Input: part model. Units: mm. Frame: model coordinates. Round coordinates to 2 decimals unless told otherwise and drop trailing zeros. Loops run counter-clockwise (first coordinate to the right, second up) from the corner with the lowest first, then second, coordinate; pieces in that order, holes last.
1) Ray query, line 1 along Y through (x, z) = (-118.6, 5.15); line 2 along Y through (x, z) = (-121.85, 5.8). Return the intervals inside material, ascending.
2) Section B-B, the plane x = -120.2. State how many separate pieces and enclosed holes the cut face has, and give its area (3 significant figures).
3) Section A-A, the plane y = 80. Return loops of the section in (x, z), and give its area (3 significant figures).
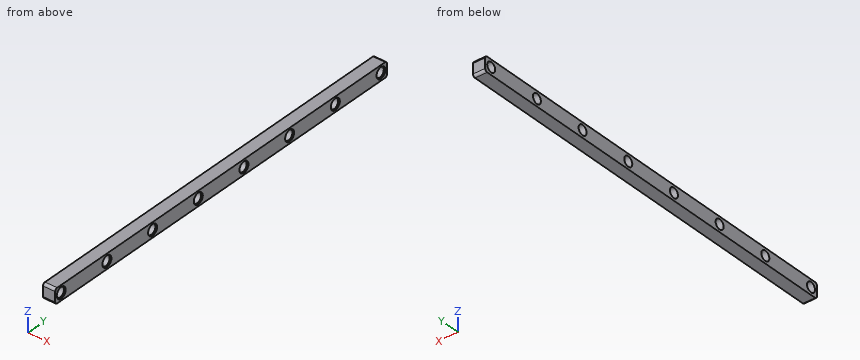
Autodesk Inventor part; units mm, degrees
ref_plane "YZ Plane" through (0, 0, 0) normal (1, 0, 0) x (0, 1, 0)
ref_plane "XZ Plane" through (0, 0, 0) normal (0, 1, 0) x (-1, 0, 0)
ref_plane "XY Plane" through (0, 0, 0) normal (0, 0, 1) x (1, 0, 0)
ref_plane "Work Plane1" through (-122.5, -83, 0) normal (1, 0, 0) x (0, -1, 0)
sketch "Sketch1" plane through (-122.5, -83, 0) normal (1, 0, 0) x (0, -1, 0)
  circle A0 centre (-140.1429, -3) radius 1.8
  circle A1 centre (-94.4286, -3) radius 1.8
  circle A2 centre (-48.7143, -3) radius 1.8
  circle A3 centre (-3, -3) radius 1.8
  circle A4 centre (-25.8571, -3) radius 1.8
  circle A5 centre (-71.5714, -3) radius 1.8
  circle A6 centre (-117.2857, -3) radius 1.8
  circle A7 centre (-163, -3) radius 1.8
  line L0 (-166, -6) -> (0, -6)
  line L1 (0, 0) -> (0, -6)
  line L2 (-166, 0) -> (0, 0)
  line L3 (-166, -6) -> (-166, 0)
  point P0 (-83, 0)
extrude "Extrusion1" add sketch "Sketch1" along normal blind 5
fillet "Fillet1" radius 1 4 edges at (-120, -83, 0) (-120, -83, 6) (-120, 83, 6) (-120, 83, 0)
sketch "Sketch2" plane through (-117.5, -83, 0) normal (1, 0, 0) x (0, 0, -1)
  arc A0 (0, 165) -> (-1, 166) centre (-1, 165) ccw
  line L0 (-1, 166) -> (-5, 166)
  arc A1 (-5, 166) -> (-6, 165) centre (-5, 165) ccw
  line L1 (-6, 165) -> (-6, 1)
  arc A2 (-6, 1) -> (-5, 0) centre (-5, 1) ccw
  line L2 (-5, 0) -> (-1, 0)
  arc A3 (-1, 0) -> (0, 1) centre (-1, 1) ccw
  line L3 (0, 1) -> (0, 165)
  circle A4 centre (-3, 163) radius 1.8
  circle A5 centre (-3, 117.2857) radius 1.8
  circle A6 centre (-3, 71.5714) radius 1.8
  circle A7 centre (-3, 25.8571) radius 1.8
  circle A8 centre (-3, 3) radius 1.8
  circle A9 centre (-3, 48.7143) radius 1.8
  circle A10 centre (-3, 94.4286) radius 1.8
  circle A11 centre (-3, 140.1429) radius 1.8
  point P0 (0, 83)
hole "Hole1" at (-117.5, -80, 3) at (-117.5, -57.1429, 3) at (-117.5, -34.2857, 3) at (-117.5, -11.4286, 3) at (-117.5, 11.4286, 3) at (-117.5, 34.2857, 3) at (-117.5, 57.1429, 3) at (-117.5, 80, 3) direction (-1, 0, 0) diameter 4 end through all counterbore diameter 4.5 counterbore depth 0.5
properties part number "petg_holder"
Final values:
1. line 1: y = -82.99 to 82.99
1. line 2: y = -82.6 to 82.6
2. separate pieces: 1
2. enclosed holes: 8
2. area: 895 mm2
3. outline: (-122.5, 0) - (-117.5, 0) - (-117.5, 0.75) - (-118, 0.75) - (-118, 1) - (-122.5, 1) - close; (-122.5, 5) - (-118, 5) - (-118, 5.25) - (-117.5, 5.25) - (-117.5, 6) - (-122.5, 6) - close
3. area: 9.75 mm2
